from build123d import *

# Parameters (mm, degrees)
F0_W     = 127.76
F0_H     = 85.48
F1_DEPTH = 8
F3_W     = 124.36
F3_H     = 82.08
F4_DEPTH = 8
F5_SIZE  = 8
F6_R     = 3
F7_R     = 5.125
F8_DEPTH = 10


with BuildPart() as f1:
    # F0 (on Top) → F1 (new body)
    with BuildSketch(Plane.XY):
        Rectangle(F0_W, F0_H)
    extrude(amount=F1_DEPTH)

    # F3 (on face) → F4 (join)
    with BuildSketch(Plane.XY.offset(8)):
        Rectangle(F3_W, F3_H)
    extrude(amount=F4_DEPTH)

    # F5
    f5_edges = [f1.edges().sort_by_distance(p)[0] for p in [
        (-62.18, 41.04, 12),
    ]]
    chamfer(f5_edges, length=F5_SIZE)

    # F6
    f6_edges = [f1.edges().sort_by_distance(p)[0] for p in [
        (-63.88, 42.74, 4),
        (-63.88, -42.74, 4),
        (63.88, -42.74, 4),
        (63.88, 42.74, 4),
        (-62.18, 33.04, 12),
        (-62.18, -41.04, 12),
        (62.18, -41.04, 12),
        (62.18, 41.04, 12),
        (-54.18, 41.04, 12),
    ]]
    fillet(f6_edges, radius=F6_R)

    # F7 (on face) → F8 (cut)
    with BuildSketch(Plane(origin=(0, 0, 0), x_dir=(1, 0, 0), z_dir=(0, 0, -1))):
        Circle(F7_R)
        with Locations((48.88, 27.74)):
            Circle(F7_R)
        with Locations((48.88, -27.74)):
            Circle(F7_R)
        with Locations((-48.88, -27.74)):
            Circle(F7_R)
        with Locations((-48.88, 27.74)):
            Circle(F7_R)
    extrude(amount=-F8_DEPTH, mode=Mode.SUBTRACT)


solid = f1.part
Source: CAD feature listing. Evaluate the final solid. Frame: model axes, mm. A direction names the side the tool comes from. Give positions to 0.01 mm unless a question says otherwise; leave off trailing zeros. Write each loop counter-clockwise with the first axis right and the second up, starting at its lowest first coordinate (ties: lowest second). Pieces come first, ordered by that corner, then holes. Notation, with made-up numbers: M 37.25,57 L 46.25,57 A13 ccw 46.25,82 Z; hole C -21.75,-6.75 d4. An arc over 180 degrees is marked long. Return JSON: item names as keys, results as strings. Group by question number.
1) Draft query along X for faces 5 (the face through (61.28, 40.18, 12.06)), 6 (the face through (2, 41.04, 12)), 7 (the face through (53.77, 26.2, 4.93)), 8 (the face through (-1.111, 5.003, 4.93)). Return one class per face: released by +X, released by -X, zero draft, split by the parting line, or undercut.
2) Ray query, L1, parallel to X at y = 27.74, z = 2.75 (3 decimals); L2, parallel to Y at x = -48.88, z = 4.25 (3 decimals); L3, parallel to X at y = 31, z = 14.5. Return the intervals inside material, ascending.
3) Cut plane A-A, the plane z = 4. Output: boundary loops of the cut face in (x, y) (3 decimals).
4) Set-up query: faces 1 (the face through (-61.32, -40.14, 12.06)), 2 (the face through (-58.22, 37, 11.94)), 3 (the face through (-49, -28, 10)), 4 (the face through (61.32, -40.14, 12.06)). Return all of +Z, -Z, +X, -X, +Y, -Y with unobstructed straight access to the full face (end or side cutting, diameter ignored); none if empty.
5) Cut plane C-C, the plane x = 0. Output: boundary loops of the cut face in (y, z) (3 decimals), then the cut area to 3 significant figures.
6) Cut plane D-D, the plane x = -21.5. Output: boundary loops of the cut face in (y, z), then the cut area to 3 significant figures.
7) Cut plane B-B, the plane y = 36. Output: boundary loops of the cut face in (x, z).
8) First-contact query: pin 1 Ø3 at (x, y) = (-47, -27) entering from -Z; pin 2 Ø9 at (y, z) = (0.5, 10.5) entering from -X; pin 3 Ø2 at (x, z) = (-12, 11.5) entering from +Y; pin 4 Ø4 at (x, z) = (-3, 13.5) entering from -Y. Flat tips, straight axial feed; report the tip coordinate or a pass-through.
Data:
{
 "1": {"face 5": "released by +X", "face 6": "zero draft", "face 7": "undercut", "face 8": "undercut"},
 "2": {"L1": "x = -63.88 to -54.005, -43.755 to 43.755, 54.005 to 63.88", "L2": "y = -42.74 to -32.865, -22.615 to 22.615, 32.865 to 42.74", "L3": "x = -62.18 to 62.18"},
 "3": {"outline": "M -63.88,-39.74 A3 ccw -60.88,-42.74 L 60.88,-42.74 A3 ccw 63.88,-39.74 L 63.88,39.74 A3 ccw 60.88,42.74 L -60.88,42.74 A3 ccw -63.88,39.74 Z; hole C -48.88,-27.74 d10.25; hole C -48.88,27.74 d10.25; hole C 0,0 d10.25; hole C 48.88,-27.74 d10.25; hole C 48.88,27.74 d10.25"},
 "4": {"face 1": "+Z, -X, -Y", "face 2": "+Z, -X, +Y", "face 3": "-Z", "face 4": "+Z, +X, -Y"},
 "5": {"outline": "M -42.74,0 L -5.125,0 L -5.125,10 L 5.125,10 L 5.125,0 L 42.74,0 L 42.74,8 L 41.04,8 L 41.04,16 L -41.04,16 L -41.04,8 L -42.74,8 Z", "area": "1,240 mm²"},
 "6": {"outline": "M -42.74,0 L 42.74,0 L 42.74,8 L 41.04,8 L 41.04,16 L -41.04,16 L -41.04,8 L -42.74,8 Z", "area": "1,340 mm²"},
 "7": {"outline": "M -63.88,0 L 63.88,0 L 63.88,8 L 62.18,8 L 62.18,16 L -59.22,16 L -59.22,8 L -63.88,8 Z"},
 "8": {"pin 1": "stops at z = 10", "pin 2": "stops at x = -63.88", "pin 3": "stops at y = 41.04", "pin 4": "stops at y = -41.04"}
}
